```python
from build123d import *

# Parameters (mm, degrees)
EXTRUDE_1_DEPTH       = 330
EXTRUDE_3_DEPTH       = 330
PATTERN_CURVE_1_COUNT = 11
PATTERN_CURVE_1_PITCH = 10
SKETCH_3_R            = 2.25
CUT_EXTRUDE_1_DEPTH   = 6
SKETCH_4_R            = 1.6
SKETCH_4_R_2          = 2.1
SKETCH_4_R_3          = 2.5
SKETCH_4_R_4          = 2.6
SKETCH_4_R_5          = 1.1
CUT_EXTRUDE_2_DEPTH   = 6


with BuildPart() as part:
    # Эскиз1 → Вытянуть1 (new body)
    with BuildSketch(Plane.XY):
        with BuildLine():
            Line((0, 40), (1.528979332, 40))
            ThreePointArc((1.528979332, 40), (2.225614441, 39.717425624), (2.528547087, 39.029399052))
            Line((2.528547087, 39.029399052), (3.5, 6))
            Line((3.5, 6), (118.5, 6))
            Line((118.5, 6), (119.471452913, 39.029399052))
            ThreePointArc((119.471452913, 39.029399052), (119.774385559, 39.717425624), (120.471020668, 40))
            Line((120.471020668, 40), (122, 40))
            Line((122, 40), (122, 0))
            Line((122, 0), (0, 0))
            Line((0, 0), (0, 40))
        make_face()
    extrude(amount=EXTRUDE_1_DEPTH)

    # Эскиз2 → Вытянуть3 (add)
    with BuildSketch(Plane.XY.offset(330)):
        with BuildLine():
            Line((10.5, 39.5), (9.25, 6))
            Line((9.25, 6), (12.75, 6))
            Line((12.75, 6), (11.5, 39.5))
            ThreePointArc((11.5, 39.5), (11, 40), (10.5, 39.5))
        make_face()
    extrude_3 = extrude(amount=-EXTRUDE_3_DEPTH)

    # Кривая1: Вытянуть3 ×11
    with Locations(*[(i * PATTERN_CURVE_1_PITCH, 0, 0) for i in range(1, PATTERN_CURVE_1_COUNT)]):
        add(extrude_3)

    # Эскиз3 → Вырез-Вытянуть1 (cut)
    with BuildSketch(Plane.XZ):
        with Locations((28, 322)):
            Circle(SKETCH_3_R)
        with Locations((94, 322)):
            Circle(SKETCH_3_R)
        with Locations(Location((94, 8, 0), (0, 0, 236.251011404))):
            Circle(SKETCH_3_R)
        with Locations(Location((28, 8, 0), (0, 0, 56.251011404))):
            Circle(SKETCH_3_R)
    extrude(amount=-CUT_EXTRUDE_1_DEPTH, mode=Mode.SUBTRACT)

    # Эскиз4 → Вырез-Вытянуть2 (cut)
    with BuildSketch(Plane(origin=(1.487985642, 0, 27.400529356), x_dir=(1, 0, 0), z_dir=(0, -1, 0))):
        with Locations((75.912014358, 233.599470644)):
            Circle(SKETCH_4_R)
        with Locations((59.512014358, 123.599470644)):
            Circle(SKETCH_4_R)
        with Locations((75.912014358, 200.099470644)):
            Circle(SKETCH_4_R)
        with Locations((28.512014358, 276.599470644)):
            Circle(SKETCH_4_R)
        with Locations((28.512014358, 156.599470644)):
            Circle(SKETCH_4_R)
        with Locations((59.512014358, 13.599470644)):
            Circle(SKETCH_4_R)
        with Locations((38.512014358, 113.599470644)):
            Circle(SKETCH_4_R_2)
        with Locations((65.832014358, 79.479470644)):
            Circle(SKETCH_4_R_3)
        with Locations((100.512014358, 251.599470644)):
            Circle(SKETCH_4_R_4)
        with Locations((85.842014358, 140.399470644)):
            Circle(SKETCH_4_R_5)
    extrude(amount=-CUT_EXTRUDE_2_DEPTH, mode=Mode.SUBTRACT)


solid = part.part
```
Could you check a few things on this model? Use its own coordinates, in mm. A direction names the side the tool comes from. Round coordinates to 2 decimals unless told otherwise and drop trailing zeros.
Q1. Thinking about a two-plate mould opening in X: for faces 3 (the flat face through (112.134, 22.516, 167.31)), 4 (the flat face through (62, 0, 163)), 5 (the flat face through (36, 6, 163)), 6 (the flat face through (122, 20, 163)), which applies, pulls with the +X half, pulls with the -X half, needs draft (parallel to the pull), parting line crosses it, or undercut?
Q2. On a 3-axis mill with a long thin cutter (end or side, diameter ignored), from which of +Z, -Z, +X, -X, +Y, -Y can I reach the whole of each face in a straight line? I mean faces 1 (the flat face through (32.134, 22.516, 167.31)), 2 (the flat face through (61, 13, 0)). Say none if no direction works.
Q3. For P1, Ø1.9, axis at x = 30, z = 304, coming from the +Y side; P2, Ø2, axis at x = 105.5, z = 112.5, coming from the +Y side; P3, Ø1.6, axis at x = 61, z = 40.5, coming from the -Y side, each with a flat end and sliding along its axis, tell me the tip position at first contact or that it passes through.
Q4. Please list where these lines run through material, in increasing order: L1, parallel to X at y = 4.4, z = 322; L2, parallel to Z at x = 77.4, y = 3.1; L3, parallel to X at y = 3.9, z = 184.
Q5. I want a section at A-A (y = 15.5). Give the number of separate pieces and of enclosed holes in the cut face, and give its area (3 significant figures).
Answer below:
1. face 3: undercut
1. face 4: needs draft
1. face 5: undercut
1. face 6: pulls with the +X half
2. face 1: +Z, -Z, +Y
2. face 2: -Z, +X, -X, +Y, -Y
3. P1: stops at y = 40
3. P2: stops at y = 6
3. P3: stops at y = 6
4. L1: x = 0 to 25.75, 30.25 to 91.75, 96.25 to 122
4. L2: z = 0 to 225.9, 229.1 to 259.4, 262.6 to 330
4. L3: x = 0 to 28.4, 31.6 to 122
5. separate pieces: 13
5. enclosed holes: 0
5. area: 12,300 mm2
